from build123d import *

# Parameters (mm, degrees)
SKETCH_1_W      = 27.3
SKETCH_1_H      = 27.8
EXTRUDE_1_DEPTH = 1.6
SKETCH_2_W      = 21.7
SKETCH_2_H      = 19.268
EXTRUDE_2_DEPTH = 1.5
SKETCH_3_W      = 21.744
SKETCH_3_H      = 10.864
EXTRUDE_3_DEPTH = 0.1


with BuildPart() as part:
    # 草图1 → 凸台-拉伸1 (new body)
    with BuildSketch(Plane.XY):
        Rectangle(SKETCH_1_W, SKETCH_1_H)
    extrude(amount=EXTRUDE_1_DEPTH)

    # 草图2 → 凸台-拉伸2 (add)
    with BuildSketch(Plane.XY.offset(1.6)):
        Rectangle(SKETCH_2_W, SKETCH_2_H)
    extrude(amount=EXTRUDE_2_DEPTH)

    # 草图3 → 凸台-拉伸3 (add)
    with BuildSketch(Plane.XY.offset(3.1)):
        with Locations((0, 2.102)):
            Rectangle(SKETCH_3_W, SKETCH_3_H)
    extrude(amount=EXTRUDE_3_DEPTH)


solid = part.part
Build history of the part. All positions in model axes, mm. A direction names the side the tool comes from. Round coordinates to 2 decimals unless told otherwise and drop trailing zeros. Write each loop counter-clockwise with the first axis right and the second up, starting at its lowest first coordinate (ties: lowest second). Pieces come first, ordered by that corner, then holes. Notation, with made-up numbers: (-33, 62.5) -> (-17, 62.5) arc R27 ccw to (-17, 98.5) -> close; hole circle Ø3 at (11, 25.5). An arc over 180 degrees is marked (long way). Use one line per item in the form item = value.
Q1. Band-saw the part on C-C, the plane z = 2.65. Write the cut outline in (x, y), then the cut area to 3 significant figures.
Conclusion:
outline = (-10.85, -9.63) -> (10.85, -9.63) -> (10.85, 9.63) -> (-10.85, 9.63) -> close
area = 418 mm²
Q2. Tool access for faces 1 (the flat face through (0, -9.634, 2)), 2 (the flat face through (-13.65, 0, 1)), 3 (the flat face through (0, 9.634, 2)): list every direction of +Z, -Z, +X, -X, +Y, -Y with a clear straight run to the whole face (end or side of a thin tool).
Conclusion:
face_1 = +Z, +X, -X, -Y
face_2 = +Z, -Z, -X, +Y, -Y
face_3 = +Z, +X, -X, +Y
Q3. Drill centre lines: L1, parallel to Z at x = 5.25, y = -3.5; L2, parallel to Z at x = 11, y = -0.5; L3, parallel to Y at x = -7, z = 2.55. Where is each one in solid material? Low to high.
Conclusion:
L1 = 0 to 3.1
L2 = 0 to 1.6
L3 = -9.63 to 9.63
Q4. Band-saw the part on D-D, the plane x = -11.5. Write the cut outline in (y, z), then the cut area to 3 significant figures.
Conclusion:
outline = (-13.9, 0) -> (13.9, 0) -> (13.9, 1.6) -> (-13.9, 1.6) -> close
area = 44.5 mm²
Q5. Band-saw the part on A-A, the plane x = 6. Write the cut outline in (y, z), then the cut area to 3 significant figures.
Conclusion:
outline = (-13.9, 0) -> (13.9, 0) -> (13.9, 1.6) -> (9.63, 1.6) -> (9.63, 3.1) -> (7.53, 3.1) -> (7.53, 3.2) -> (-3.33, 3.2) -> (-3.33, 3.1) -> (-9.63, 3.1) -> (-9.63, 1.6) -> (-13.9, 1.6) -> close
area = 74.5 mm²
Q6. Drop flat-ended pins along their axis: P1, Ø2.5, axis at x = -0.5, y = 9, coming from the +Z side; P2, Ø1, axis at y = -9.5, z = 2.5, coming from the +X side. Give the stop position or say it passes through.
Conclusion:
P1 = 3.1
P2 = 10.85
